For this review, take the finished solid that the model builds, in its own axes (mm). A direction names the side the tool comes from. Coordinates: 2 decimals unless noted, no trailing zeros. Order: outer loops, then holes, each group sorted by start corner. A loop starts at its lowest first (then second) coordinate and runs counter-clockwise, first axis right, second up. Notation, with made-up numbers: (46, 66.5) -> (91, 66.5) arc R11 ccw to (91, 70.5) -> close; hole circle Ø11 at (87, 5). An arc over 180 degrees is marked (long way). Answer as a JSON object with one key per item and string values. Group by question number.
1) Add section C-C, the plane y = -116. Write out the cut boundary in (x, z).
2) For pin 1 (2.5 mm diameter, centred on y = -50, z = 0, fed in from -X); pin 2 (1 mm diameter, centred on x = 3, z = 7, fed in from +Y), all flat-tipped, find the tip position at first contact; note any pin that passes through.
3) Wall thickness on L1, parallel to Y at x = 3.65, z = 10; L2, parallel to Y at x = 0.3, z = 15; L3, parallel to Z at x = 0.6, y = -175.5: over which ranges is each line inside the solid? List them lowest first.
4) Add section B-B, the plane x = 1.75. Count the separate pieces of the cut face and the enclosed holes in it, then the cut area to 3 significant figures.
5) Machinability: for faces 4 (the cylindrical face through (2, 10.4, 33)), 5 (the flat face through (1.97, -68.16, -25.13)), which of the approach directions +Z, -Z, +X, -X, +Y, -Y give a long, thin tool a straight path to every point of the face, cutting with its end or side? Answer none if there is none.
6) Draft analysis for pull direction Z (two halves, no side actions). For faces 1 (the cylindrical face through (1.972, -186.907, -1.534)), 2 (the flat face through (4, -79, 6)), 3 (the flat face through (1.972, -103.343, 31.043)), state which applies: +Z half, -Z half, draft (parallel to the pull), parting line (faces both ways), or undercut.
7) Add section A-A, the plane z = 28. Write out the cut boundary in (x, y), then the cut area to 3 significant figures.
8) Add section D-D, the plane y = -163. Write out the cut boundary in (x, z), then the cut area to 3 significant figures.
from build123d import *

# Parameters (mm, degrees)
SKETCH_1_R               = 41.5
SKETCH_1_R_2             = 23
EXTRUDE_1_DEPTH          = 4
SKETCH_3_R               = 34.6
SKETCH_3_R_2             = 7.075
CUT_EXTRUDE_2_DEPTH      = 5
SKETCH_2_R               = 1.6
CUT_EXTRUDE_1_DEPTH      = 5
PATTERN_CIRCULAR_1_COUNT = 12
FILLET_1_R               = 50
SKETCH_4_R               = 1.55
CUT_EXTRUDE_3_DEPTH      = 10
SKETCH_5_R               = 1.6
EXTRUDE_2_DEPTH          = 4
FILLET_2_R               = 20
SKETCH_6_R               = 1.55
CUT_EXTRUDE_4_DEPTH      = 10
FILLET_3_R               = 35
SKETCH_7_R               = 1.4
CUT_EXTRUDE_5_DEPTH      = 10
SKETCH_8_R               = 1.35
CUT_EXTRUDE_6_DEPTH      = 10


with BuildPart() as part:
    # 草图1 → 凸台-拉伸1 (new body)
    with BuildSketch(Plane(origin=(0, 0, 0), x_dir=(0, 0, -1), z_dir=(1, 0, 0))):
        Circle(SKETCH_1_R)
        with BuildLine():
            Line((1.96511799, -157.084103524), (40.159775356, -10.461474243))
            ThreePointArc((40.159775356, -10.461474243), (-3.1483436, -41.380405177), (-41.280230201, -4.265277778))
            Line((-41.280230201, -4.265277778), (-22.878199871, -182.363888889))
            ThreePointArc((-22.878199871, -182.363888889), (-16.404454744, -163.87877596), (1.96511799, -157.084103524))
        make_face()
        with Locations((0, -180)):
            Circle(SKETCH_1_R_2)
    extrude(amount=EXTRUDE_1_DEPTH)

    # 草图3 → 切除-拉伸2 (cut)
    with BuildSketch(Plane.ZY):
        Circle(SKETCH_3_R)
        with Locations((0, -180)):
            Circle(SKETCH_3_R_2)
    extrude(amount=-CUT_EXTRUDE_2_DEPTH, mode=Mode.SUBTRACT)

    # 草图2 → 切除-拉伸1 (cut)
    with BuildSketch(Plane.ZY):
        with Locations((0, 37)):
            Circle(SKETCH_2_R)
    cut_extrude_1 = extrude(amount=-CUT_EXTRUDE_1_DEPTH, mode=Mode.SUBTRACT)

    # 阵列(圆周)1: 切除-拉伸1 ×12 about axis
    pattern_circular_1_axis = Axis((0, 0, 0), (1, 0, 0))
    for i in range(1, PATTERN_CIRCULAR_1_COUNT):
        add(cut_extrude_1.rotate(pattern_circular_1_axis, i * 360 / PATTERN_CIRCULAR_1_COUNT), mode=Mode.SUBTRACT)

    # 圆角1
    fillet_1_edges = [part.edges().sort_by_distance(p)[0] for p in [
        (2, -157.084103524, -1.96511799),
    ]]
    fillet(fillet_1_edges, radius=FILLET_1_R)

    # 草图4 → 切除-拉伸3 (cut)
    with BuildSketch(Plane(origin=(4, 0, 0), x_dir=(0, 0, -1), z_dir=(1, 0, 0))):
        with Locations((22.71706237, -57.586327173)):
            Circle(SKETCH_4_R)
        with Locations((10.112876536, -105.971598687)):
            Circle(SKETCH_4_R)
    extrude(amount=-CUT_EXTRUDE_3_DEPTH, mode=Mode.SUBTRACT)

    # 草图5 → 凸台-拉伸2 (add)
    with BuildSketch(Plane(origin=(4, 0, 0), x_dir=(0, 0, -1), z_dir=(1, 0, 0))):
        with BuildLine():
            Line((-41.306779105, 4), (-49, 4))
            ThreePointArc((-49, 4), (-53, 0), (-49, -4))
            Line((-49, -4), (-41.306779105, -4))
            ThreePointArc((-41.306779105, -4), (-41.5, 0), (-41.306779105, 4))
        make_face()
        with Locations((-49, 0)):
            Circle(SKETCH_5_R, mode=Mode.SUBTRACT)
    extrude(amount=-EXTRUDE_2_DEPTH)

    # 圆角2
    fillet_2_edges = [part.edges().sort_by_distance(p)[0] for p in [
        (2, 4, 41.306779105),
    ]]
    fillet(fillet_2_edges, radius=FILLET_2_R)

    # 草图6 → 切除-拉伸4 (cut)
    with BuildSketch(Plane(origin=(4, 0, 0), x_dir=(0, 0, -1), z_dir=(1, 0, 0))):
        with Locations((0, -50)):
            Circle(SKETCH_6_R)
        with Locations((-1.746038475, -130)):
            Circle(SKETCH_6_R)
    extrude(amount=-CUT_EXTRUDE_4_DEPTH, mode=Mode.SUBTRACT)

    # 圆角3
    fillet_3_edges = [part.edges().sort_by_distance(p)[0] for p in [
        (2, -4, 41.306779105),
    ]]
    fillet(fillet_3_edges, radius=FILLET_3_R)

    # 草图7 → 切除-拉伸5 (cut)
    with BuildSketch(Plane(origin=(4, 0, 0), x_dir=(0, 0, -1), z_dir=(1, 0, 0))):
        with Locations((-1.493538323, -61.450142252)):
            Circle(SKETCH_7_R)
        with Locations((20.236020893, -67.110612761)):
            Circle(SKETCH_7_R)
        with Locations((-8.425840532, -88.062041585)):
            Circle(SKETCH_7_R)
        with Locations((13.303718684, -93.722512094)):
            Circle(SKETCH_7_R)
    extrude(amount=-CUT_EXTRUDE_5_DEPTH, mode=Mode.SUBTRACT)

    # 草图8 → 切除-拉伸6 (cut)
    with BuildSketch(Plane(origin=(4, 0, 0), x_dir=(0, 0, -1), z_dir=(1, 0, 0))):
        with Locations((-6.375878439, -60.178310552)):
            Circle(SKETCH_8_R)
        with Locations((-13.308180648, -86.790209885)):
            Circle(SKETCH_8_R)
    extrude(amount=-CUT_EXTRUDE_6_DEPTH, mode=Mode.SUBTRACT)


solid = part.part
Output values:
{
 "1": {"outline": "(0, -12.67) -> (4, -12.67) -> (4, 29.74) -> (0, 29.74) -> close"},
 "2": {"pin 1": "passes through", "pin 2": "stops at y = 40.99"},
 "3": {"L1": "y = -200.71 to -33.12, 33.12 to 40.28", "L2": "y = -197.44 to -31.18, 31.18 to 38.69", "L3": "z = -22.56 to -5.46, 5.46 to 23.59"},
 "4": {"separate pieces": "1", "enclosed holes": "25", "area": "9,540 mm²"},
 "5": {"face 4": "+X, -X", "face 5": "-Z, +X, -X"},
 "6": {"face 1": "undercut", "face 2": "draft", "face 3": "+Z half"},
 "7": {"outline": "(0, -132.79) -> (4, -132.79) -> (4, -20.33) -> (0, -20.33) -> close; (0, 20.33) -> (4, 20.33) -> (4, 30.63) -> (0, 30.63) -> close", "area": "491 mm²"},
 "8": {"outline": "(0, -16.27) -> (4, -16.27) -> (4, 24.88) -> (0, 24.88) -> close", "area": "165 mm²"}
}
